Work out the finished part from the listing and answer in its coordinate system (mm). Coordinates: 2 decimals unless noted, no trailing zeros. Order: outer loops, then holes, each group sorted by start corner. A loop starts at its lowest first (then second) coordinate and runs counter-clockwise, first axis right, second up.
1. The part is cut by section B-B, the plane z = 0.85. Give the vertices of the cut face in (x, y).
2. Find the intervals of material crossed by probe 1 along X at (y, z) = (-1, -2.15); probe 2 along Y at (x, z) = (-348.5, 0.4); probe 3 along X at (y, z) = (3.5, -1.6), in increasing order.
3. The part is cut by section A-A, the plane y = 0. Give the vertices of the cut face in (x, z), then the cut area to 3 significant figures.
```python
from build123d import *

# Parameters (mm, degrees)
PLAT_W                          = 30
PLAT_H                          = 5
EL_MENT_M_CANO_SOUD_1_DEPTH     = 817
DIAM_TRE_DU_PER_AGE_13_0_13_1_D = 13
R_P_TITION_LIN_AIRE2_COUNT      = 3
R_P_TITION_LIN_AIRE2_PITCH      = 348.5


with BuildPart() as part:
    # plat → Elément mécano-soudé1 (new body)
    with BuildSketch(Plane.YZ.offset(-408.5)):
        Rectangle(PLAT_W, PLAT_H)
    extrude(amount=EL_MENT_M_CANO_SOUD_1_DEPTH)

    # Diamètre du perçage Ø13.0 (13)1 (through all)
    with Locations(Plane(origin=(0, 0, -2.5), x_dir=(-1, 0, 0), z_dir=(0, 0, -1))):
        with Locations((348.5, 0)):
            diam_tre_du_per_age_13_0_13_1 = Hole(DIAM_TRE_DU_PER_AGE_13_0_13_1_D / 2)

    # Répétition linéaire2: Diamètre du perçage Ø13.0 (13)1 ×3
    with Locations(*[(i * R_P_TITION_LIN_AIRE2_PITCH, 0, 0) for i in range(1, R_P_TITION_LIN_AIRE2_COUNT)]):
        add(diam_tre_du_per_age_13_0_13_1, mode=Mode.SUBTRACT)


solid = part.part
```
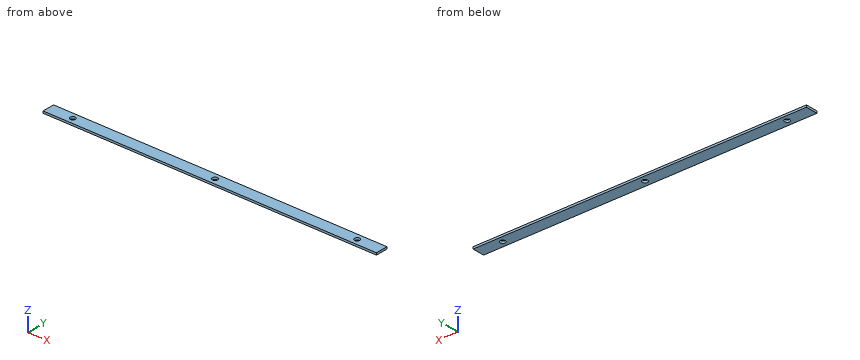
Geometry says:
1. outline: (-408.5, -15) - (408.5, -15) - (408.5, 15) - (-408.5, 15) - close; hole circle Ø13 at (-348.5, 0); hole circle Ø13 at (0, 0); hole circle Ø13 at (348.5, 0)
2. probe 1: x = -408.5 to -354.92, -342.08 to -6.42, 6.42 to 342.08, 354.92 to 408.5
2. probe 2: y = -15 to -6.5, 6.5 to 15
2. probe 3: x = -408.5 to -353.98, -343.02 to -5.48, 5.48 to 343.02, 353.98 to 408.5
3. outline: (-408.5, -2.5) - (-355, -2.5) - (-355, 2.5) - (-408.5, 2.5) - close; (-342, -2.5) - (-6.5, -2.5) - (-6.5, 2.5) - (-342, 2.5) - close; (6.5, -2.5) - (342, -2.5) - (342, 2.5) - (6.5, 2.5) - close; (355, -2.5) - (408.5, -2.5) - (408.5, 2.5) - (355, 2.5) - close
3. area: 3,890 mm2
